```python
from build123d import *

# Parameters (mm, degrees)
BLANKSKE_W             = 25
BLANKSKE_H             = 5.7
BLANK_DEPTH            = 3
TOOTHCUTSIM_DEPTH      = 26.816467613
TEETHCUTS_COUNT        = 12
TEETHCUTS_PITCH        = 2.199114855
MIRROR_2_COPY_1_DEPTH  = 26.816467613
MIRROR_2_COPY_2_DEPTH  = 26.816467613
MIRROR_2_COPY_3_DEPTH  = 26.816467613
MIRROR_2_COPY_4_DEPTH  = 26.816467613
MIRROR_2_COPY_5_DEPTH  = 26.816467613
MIRROR_2_COPY_6_DEPTH  = 26.816467613
MIRROR_2_COPY_7_DEPTH  = 26.816467613
MIRROR_2_COPY_8_DEPTH  = 26.816467613
MIRROR_2_COPY_9_DEPTH  = 26.816467613
MIRROR_2_COPY_10_DEPTH = 26.816467613
MIRROR_2_COPY_11_DEPTH = 26.816467613
CUT_EXTRUDE_2_DEPTH    = 26.816467613
FILLET_1_R             = 0.2
FILLET_2_R             = 0.2
FILLET_3_R             = 0.2
SKETCH_2_R             = 1.5
EXTRUDE_1_DEPTH        = 1.5
SKETCH_3_R             = 0.5
CUT_EXTRUDE_3_DEPTH    = 27.033440034


with BuildPart() as part:
    # BlankSke → Blank (new body)
    with BuildSketch(Plane.XY):
        with Locations((12.5, 2.85)):
            Rectangle(BLANKSKE_W, BLANKSKE_H)
    blank = extrude(amount=-BLANK_DEPTH)

    # TooCutSkeSim → ToothCutSim (cut, through all)
    with BuildSketch(Plane.XY):
        Polygon((0.404488327, 4.125), (-0.404488327, 4.125), (-0.818379909, 5.7254), (0.818379909, 5.7254), align=None)
    toothcutsim = extrude(amount=-TOOTHCUTSIM_DEPTH, mode=Mode.SUBTRACT)

    # TeethCuts: ToothCutSim ×12
    with Locations(*[(i * TEETHCUTS_PITCH, 0, 0) for i in range(1, TEETHCUTS_COUNT)]):
        add(toothcutsim, mode=Mode.SUBTRACT)

    # 镜向2: Blank, ToothCutSim across plane
    add(blank.mirror(Plane(origin=(0, 0, -3), x_dir=(0, 0, 1), z_dir=(0, -1, 0))))
    add(toothcutsim.mirror(Plane(origin=(0, 0, -3), x_dir=(0, 0, 1), z_dir=(0, -1, 0))), mode=Mode.SUBTRACT)

    # 镜向2 copy 1 sketch → 镜向2 copy 1 (cut, through all)
    with BuildSketch(Plane(origin=(2.199114855, 0, 0), x_dir=(1, 0, 0), z_dir=(0, 0, 1))):
        Polygon((0.404488327, -4.125), (-0.404488327, -4.125), (-0.818379909, -5.7254), (0.818379909, -5.7254), align=None)
    extrude(amount=-MIRROR_2_COPY_1_DEPTH, mode=Mode.SUBTRACT)

    # 镜向2 copy 2 sketch → 镜向2 copy 2 (cut, through all)
    with BuildSketch(Plane(origin=(4.39822971, 0, 0), x_dir=(1, 0, 0), z_dir=(0, 0, 1))):
        Polygon((0.404488327, -4.125), (-0.404488327, -4.125), (-0.818379909, -5.7254), (0.818379909, -5.7254), align=None)
    extrude(amount=-MIRROR_2_COPY_2_DEPTH, mode=Mode.SUBTRACT)

    # 镜向2 copy 3 sketch → 镜向2 copy 3 (cut, through all)
    with BuildSketch(Plane(origin=(6.597344565, 0, 0), x_dir=(1, 0, 0), z_dir=(0, 0, 1))):
        Polygon((0.404488327, -4.125), (-0.404488327, -4.125), (-0.818379909, -5.7254), (0.818379909, -5.7254), align=None)
    extrude(amount=-MIRROR_2_COPY_3_DEPTH, mode=Mode.SUBTRACT)

    # 镜向2 copy 4 sketch → 镜向2 copy 4 (cut, through all)
    with BuildSketch(Plane(origin=(8.79645942, 0, 0), x_dir=(1, 0, 0), z_dir=(0, 0, 1))):
        Polygon((0.404488327, -4.125), (-0.404488327, -4.125), (-0.818379909, -5.7254), (0.818379909, -5.7254), align=None)
    extrude(amount=-MIRROR_2_COPY_4_DEPTH, mode=Mode.SUBTRACT)

    # 镜向2 copy 5 sketch → 镜向2 copy 5 (cut, through all)
    with BuildSketch(Plane(origin=(10.995574275, 0, 0), x_dir=(1, 0, 0), z_dir=(0, 0, 1))):
        Polygon((0.404488327, -4.125), (-0.404488327, -4.125), (-0.818379909, -5.7254), (0.818379909, -5.7254), align=None)
    extrude(amount=-MIRROR_2_COPY_5_DEPTH, mode=Mode.SUBTRACT)

    # 镜向2 copy 6 sketch → 镜向2 copy 6 (cut, through all)
    with BuildSketch(Plane(origin=(13.19468913, 0, 0), x_dir=(1, 0, 0), z_dir=(0, 0, 1))):
        Polygon((0.404488327, -4.125), (-0.404488327, -4.125), (-0.818379909, -5.7254), (0.818379909, -5.7254), align=None)
    extrude(amount=-MIRROR_2_COPY_6_DEPTH, mode=Mode.SUBTRACT)

    # 镜向2 copy 7 sketch → 镜向2 copy 7 (cut, through all)
    with BuildSketch(Plane(origin=(15.393803985, 0, 0), x_dir=(1, 0, 0), z_dir=(0, 0, 1))):
        Polygon((0.404488327, -4.125), (-0.404488327, -4.125), (-0.818379909, -5.7254), (0.818379909, -5.7254), align=None)
    extrude(amount=-MIRROR_2_COPY_7_DEPTH, mode=Mode.SUBTRACT)

    # 镜向2 copy 8 sketch → 镜向2 copy 8 (cut, through all)
    with BuildSketch(Plane(origin=(17.59291884, 0, 0), x_dir=(1, 0, 0), z_dir=(0, 0, 1))):
        Polygon((0.404488327, -4.125), (-0.404488327, -4.125), (-0.818379909, -5.7254), (0.818379909, -5.7254), align=None)
    extrude(amount=-MIRROR_2_COPY_8_DEPTH, mode=Mode.SUBTRACT)

    # 镜向2 copy 9 sketch → 镜向2 copy 9 (cut, through all)
    with BuildSketch(Plane(origin=(19.792033695, 0, 0), x_dir=(1, 0, 0), z_dir=(0, 0, 1))):
        Polygon((0.404488327, -4.125), (-0.404488327, -4.125), (-0.818379909, -5.7254), (0.818379909, -5.7254), align=None)
    extrude(amount=-MIRROR_2_COPY_9_DEPTH, mode=Mode.SUBTRACT)

    # 镜向2 copy 10 sketch → 镜向2 copy 10 (cut, through all)
    with BuildSketch(Plane(origin=(21.99114855, 0, 0), x_dir=(1, 0, 0), z_dir=(0, 0, 1))):
        Polygon((0.404488327, -4.125), (-0.404488327, -4.125), (-0.818379909, -5.7254), (0.818379909, -5.7254), align=None)
    extrude(amount=-MIRROR_2_COPY_10_DEPTH, mode=Mode.SUBTRACT)

    # 镜向2 copy 11 sketch → 镜向2 copy 11 (cut, through all)
    with BuildSketch(Plane(origin=(24.190263405, 0, 0), x_dir=(1, 0, 0), z_dir=(0, 0, 1))):
        Polygon((0.404488327, -4.125), (-0.404488327, -4.125), (-0.818379909, -5.7254), (0.818379909, -5.7254), align=None)
    extrude(amount=-MIRROR_2_COPY_11_DEPTH, mode=Mode.SUBTRACT)

    # 草图1 → 切除-拉伸2 (cut, through all)
    with BuildSketch(Plane.ZY):
        Polygon((0, -3), (0, 3), (-2, 3.5), (-2, -3.5), align=None)
    extrude(amount=-CUT_EXTRUDE_2_DEPTH, mode=Mode.SUBTRACT)

    # 圆角1
    fillet_1_edges = [part.edges().sort_by_distance(p)[0] for p in [
        (12.5, -3.5, -2),
    ]]
    fillet(fillet_1_edges, radius=FILLET_1_R)

    # 圆角2
    fillet_2_edges = [part.edges().sort_by_distance(p)[0] for p in [
        (12.5, 3.5, -2),
    ]]
    fillet(fillet_2_edges, radius=FILLET_2_R)

    # 圆角3
    fillet_3_edges = [part.edges().sort_by_distance(p)[0] for p in [
        (12.5, -3, 0),
        (12.5, 3, 0),
    ]]
    fillet(fillet_3_edges, radius=FILLET_3_R)

    # 草图2 → 凸台-拉伸1 (add)
    with BuildSketch(Plane(origin=(0, 0, -3), x_dir=(-1, 0, 0), z_dir=(0, 0, -1))):
        with Locations((-12.5, 0)):
            Circle(SKETCH_2_R)
    extrude(amount=EXTRUDE_1_DEPTH)

    # 草图3 → 切除-拉伸3 (cut, through all)
    with BuildSketch(Plane(origin=(0, 0, -4.5), x_dir=(-1, 0, 0), z_dir=(0, 0, -1))):
        with Locations((-12.5, 0)):
            Circle(SKETCH_3_R)
    extrude(amount=-CUT_EXTRUDE_3_DEPTH, mode=Mode.SUBTRACT)


solid = part.part
```
The model under review builds one solid part; all positions refer to its coordinate system, in mm. A direction names the side the tool comes from. Coordinates: 2 decimals unless noted, no trailing zeros. Write each loop counter-clockwise with the first axis right and the second up, starting at its lowest first coordinate (ties: lowest second). Pieces come first, ordered by that corner, then holes. Notation, with made-up numbers: (49, -9) - (105, -9) arc R34 cw to (105, 27) - close; hole circle Ø5 at (24, 66.5). An arc over 180 degrees is marked (long way). Write item = value, one per line.
(1) Consider section A-A, the plane y = 0. Give the boundary of the cut face in (x, z).
Result sheet:
outline = (0, -3) - (11, -3) - (11, -4.5) - (12, -4.5) - (12, -2) - (0, -2) - close; (13, -4.5) - (14, -4.5) - (14, -3) - (25, -3) - (25, -2) - (13, -2) - close
(2) Mouldability with a two-part tool opening along X and no side actions: class faces 4 (the face through (16.99, -4.9, -1.48)), 5 (the face through (12, -4, 0)), 6 (the face through (2.81, 4.92, -1.48)), 7 (the face through (14, 0, -4)) as pulls with the +X half, pulls with the -X half, needs draft (parallel to the pull), parting line crosses it, or undercut.
Result sheet:
face_4 = undercut
face_5 = needs draft
face_6 = undercut
face_7 = parting line crosses it
(3) Machinability: for faces 1 (the face through (6.6, -4.125, -1.5)), 2 (the face through (11.85, 0.02, -4.5)), 3 (the face through (24, 4.125, -1)), which of the approach directions +Z, -Z, +X, -X, +Y, -Y give a long, thin tool a straight path to every point of the face, cutting with its end or side? Answer none if there is none.
Result sheet:
face_1 = +Z, -Z, -Y
face_2 = -Z, +X, -X, +Y, -Y
face_3 = +Z, -Z, +Y
(4) Consider section C-C, the plane z = -3.3. Give the boundary of the cut face in (x, y), then the cut area to 3 significant figures.
Result sheet:
outline = circle Ø3 at (12.5, 0); hole circle Ø1 at (12.5, 0)
area = 6.28 mm^2
(5) For P1, Ø0.6, axis at x = 22, z = -2, coming from the -Y side (3 decimals); P2, Ø1.5, axis at x = 7, y = -0.5, coming from the +Z side; P3, Ø3.5, axis at x = 18, y = -1, coming from the -Z side, all flat-tipped, find the tip position at first contact; note any pin that passes through.
Result sheet:
P1 = -4.125
P2 = -2
P3 = -3
(6) For line 1 (Y direction, x = 13.5, z = -1.75) (1 decimal); line 2 (Y direction, x = 12.5, z = -3.4); line 3 (Z direction, x = 14.75, y = -0.75), list the stretches that pass through material, from the lowest coordinate up. Write a range as [from, to].
Result sheet:
line_1 = [-4.1, -3.4], [3.4, 4.1]
line_2 = [-1.5, -0.5], [0.5, 1.5]
line_3 = [-3, -2]
(7) Consider section D-D, the plane y = -2.25. Give the boundary of the cut face in (x, z).
Result sheet:
outline = (0, -3) - (25, -3) - (25, -2) - (0, -2) - close
